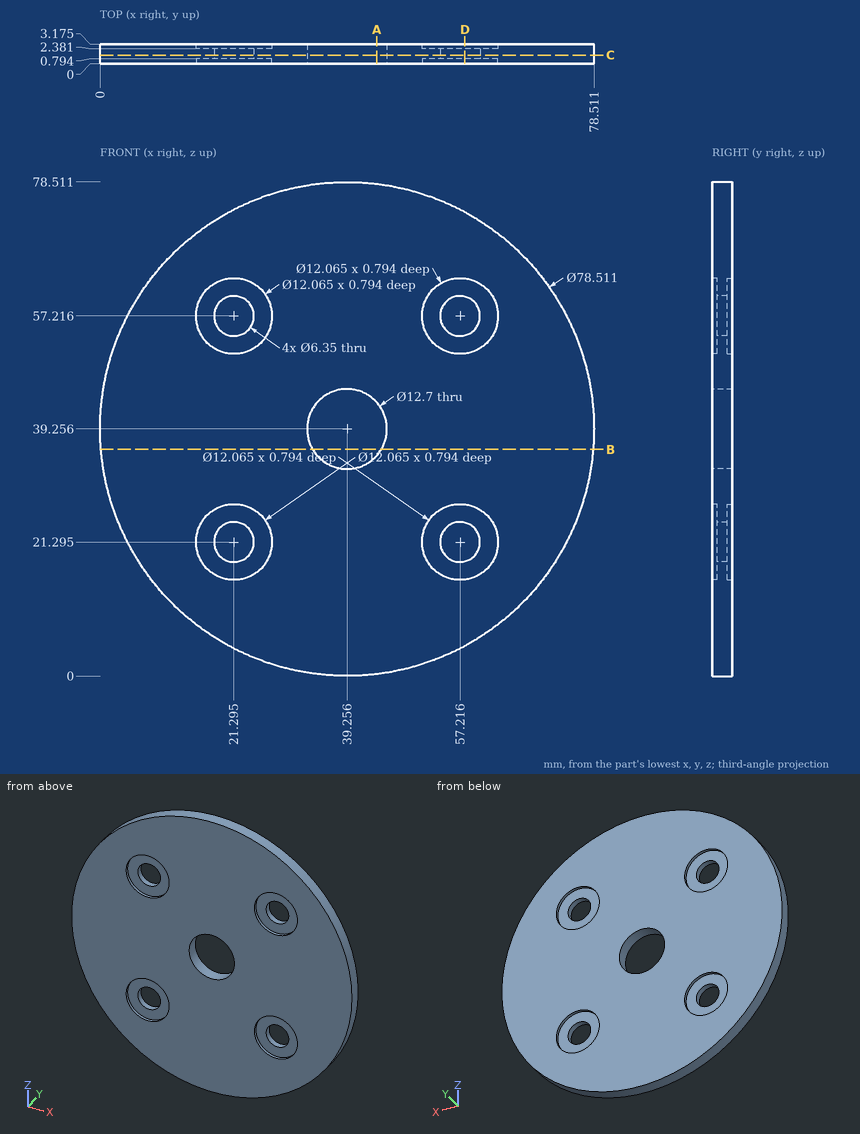
The drawing under review shows one solid part. Ordinate dimensions are in mm from its lowest x, y, z. Coordinates: 2 decimals unless noted, no trailing zeros. Loops run counter-clockwise (first coordinate to the right, second up) from the corner with the lowest first, then second, coordinate; pieces in that order, holes last.
Item 1: Add section A-A (x = 44). Write out the cut boundary in (y, z) (1 decimal), and give its area (3 significant figures).
Completed:
outline: (0, 0.3) - (3.2, 0.3) - (3.2, 35) - (0, 35) - close; (0, 43.5) - (3.2, 43.5) - (3.2, 78.2) - (0, 78.2) - close
area: 221 mm2
Item 2: Clearance check with flat-ended pins moving along their axes: pin 1 (9.5 mm diameter, centred on x = 22, z = 56, fed in from +Y) (3 decimals); pin 2 (10 mm diameter, centred on x = 57.22, z = 21.3, fed in from -Y); pin 3 (11 mm diameter, centred on x = 21.3, z = 57.22, fed in from +Y); pin 4 (3.5 mm diameter, centred on x = 57.5, z = 22.5, fed in from -Y). State where each tip first meets the part, or that it passes through.
Completed:
pin 1: stops at y = 3.175
pin 2: stops at y = 0.79
pin 3: stops at y = 2.38
pin 4: passes through
Item 3: Add section B-B (z = 36). Write out the cut boundary in (x, y) (1 decimal).
Completed:
outline: (0.1, 0) - (33.8, 0) - (33.8, 3.2) - (0.1, 3.2) - close; (44.7, 0) - (78.4, 0) - (78.4, 3.2) - (44.7, 3.2) - close
Item 4: Add section D-D (x = 58). Write out the cut boundary in (y, z) (1 decimal).
Completed:
outline: (0, 4.8) - (3.2, 4.8) - (3.2, 15.3) - (2.4, 15.3) - (2.4, 18.2) - (0.8, 18.2) - (0.8, 15.3) - (0, 15.3) - close; (0, 27.3) - (0.8, 27.3) - (0.8, 24.4) - (2.4, 24.4) - (2.4, 27.3) - (3.2, 27.3) - (3.2, 51.2) - (2.4, 51.2) - (2.4, 54.1) - (0.8, 54.1) - (0.8, 51.2) - (0, 51.2) - close; (0, 63.2) - (0.8, 63.2) - (0.8, 60.3) - (2.4, 60.3) - (2.4, 63.2) - (3.2, 63.2) - (3.2, 73.7) - (0, 73.7) - close
Item 5: Add section C-C (y = 1.4). Give the number of separate pieces and of enclosed holes in the cut face, and give its area (3 significant figures).
Completed:
separate pieces: 1
enclosed holes: 5
area: 4,590 mm2
Item 6: Wall thickness on L1, parallel to X at y = 2.2, z = 18.5 (1 decimal); L2, parallel to X at y = 1.6, z = 56; L3, parallel to Z at x = 61, y = 2.9 (1 decimal): over which ranges is each line inside the solid? List them lowest first.
Completed:
L1: x = 5.9 to 19.8, 22.8 to 55.7, 58.7 to 72.6
L2: x = 3.75 to 18.36, 24.23 to 54.28, 60.15 to 74.76
L3: z = 6.6 to 16.6, 26 to 52.5, 61.9 to 71.9
